Input: part model. Units: mm. Frame: model coordinates. Round coordinates to 2 decimals unless told otherwise and drop trailing zeros. Write each loop counter-clockwise with the first axis right and the second up, starting at its lowest first coordinate (ties: lowest second). Pieces come first, ordered by that corner, then holes. Notation, with made-up numbers: (40.25, 2.5) -> (63.25, 2.5) arc R19 cw to (63.25, 37.5) -> close; hole circle Ø1 at (32, 45). An arc over 180 degrees is marked (long way). Write item = value, one per line.
```python
from build123d import *

# Parameters (mm, degrees)
SKETCH_R        = 14
SKETCH_R_2      = 10
PAD_DEPTH       = 2
CHAMFER_SIZE    = 0.5
CHAMFER001_SIZE = 1


with BuildPart() as part:
    # Sketch → Pad (new body)
    with BuildSketch(Plane.XY):
        Circle(SKETCH_R)
        Circle(SKETCH_R_2, mode=Mode.SUBTRACT)
    extrude(amount=PAD_DEPTH)

    # Chamfer
    chamfer_edges = [part.edges().sort_by_distance(p)[0] for p in [
        (-10, 0, 2),
    ]]
    chamfer(chamfer_edges, length=CHAMFER_SIZE)

    # Chamfer001
    chamfer001_edges = [part.edges().sort_by_distance(p)[0] for p in [
        (-14, 0, 2),
    ]]
    chamfer(chamfer001_edges, length=CHAMFER001_SIZE)


solid = part.part
```
1) Line query: L1, parallel to Y at x = 0, z = 0.8; L2, parallel to X at y = -2.5, z = 0.3; L3, parallel to X at y = -6.5, z = 1.7. Output: solid intervals per line, ascending. Write a range as from..to.
Solutions:
L1 = -14..-10, 10..14
L2 = -13.77..-9.68, 9.68..13.77
L3 = -11.6..-7.86, 7.86..11.6
2) Draft query along X for faces 1 (the face through (12.932, -5.362, 0.493)), 2 (the face through (-2.17, -9.76, 0.74)), 3 (the face through (-3, 10, 0)). Return one class per face: +X half, -X half, draft (parallel to the pull), parting line (faces both ways), or undercut.
Solutions:
face_1 = parting line
face_2 = undercut
face_3 = draft
3) Cut plane C-C (z = 0.6). Return the cut outline in (x, y).
Solutions:
outline = circle Ø28 at (0, 0); hole circle Ø20 at (0, 0)
4) Cut plane A-A (x = 0). Return the cut outline in (y, z), and give its area (4 significant figures).
Solutions:
outline = (-14, 0) -> (-10, 0) -> (-10, 1.5) -> (-10.5, 2) -> (-13, 2) -> (-14, 1) -> close; (10, 0) -> (14, 0) -> (14, 1) -> (13, 2) -> (10.5, 2) -> (10, 1.5) -> close
area = 14.75 mm^2
5) First-contact query: P1, Ø1, axis at x = -8.5, z = 1, coming from the +Y side. Flat tip, straight axial feed; report the tip coordinate or a pass-through.
Solutions:
P1 = 11.49
